```python
from build123d import *

# Parameters (mm, degrees)
F0_W     = 295.148
F0_H     = 402.59
F0_R     = 6.0071
F1_DEPTH = 2.54


with BuildPart() as f1:
    # F0 (on Front) → F1 (new body)
    with BuildSketch(Plane.XZ):
        with Locations((110.562274, -122.229906)):
            Rectangle(F0_W, F0_H)
        with Locations((-24.654626, -284.789906)):
            Circle(F0_R, mode=Mode.SUBTRACT)
        with BuildLine():
            Line((-30.661726, -258.754906), (4.898274, -258.754906))
            Line((4.898274, -258.754906), (4.898274, -310.824906))
            Line((4.898274, -310.824906), (-30.661726, -310.824906))
            Line((-30.661726, -310.824906), (-30.661726, -297.489906))
            Line((-30.661726, -297.489906), (-24.654626, -297.489906))
            ThreePointArc((-24.654626, -297.489906), (-11.954626, -284.789906), (-24.654626, -272.089906))
            Line((-24.654626, -272.089906), (-30.661726, -272.089906))
            Line((-30.661726, -272.089906), (-30.661726, -258.754906))
        make_face(mode=Mode.SUBTRACT)
        with Locations((-24.654626, -183.189906)):
            Circle(F0_R, mode=Mode.SUBTRACT)
        with BuildLine():
            Line((-30.661726, -157.154906), (4.898274, -157.154906))
            Line((4.898274, -157.154906), (4.898274, -209.224906))
            Line((4.898274, -209.224906), (-30.661726, -209.224906))
            Line((-30.661726, -209.224906), (-30.661726, -195.889906))
            Line((-30.661726, -195.889906), (-24.654626, -195.889906))
            ThreePointArc((-24.654626, -195.889906), (-11.954626, -183.189906), (-24.654626, -170.489906))
            Line((-24.654626, -170.489906), (-30.661726, -170.489906))
            Line((-30.661726, -170.489906), (-30.661726, -157.154906))
        make_face(mode=Mode.SUBTRACT)
        with BuildLine():
            Line((251.786274, -290.504906), (216.226274, -290.504906))
            Line((216.226274, -290.504906), (216.226274, -238.434906))
            Line((216.226274, -238.434906), (251.786274, -238.434906))
            Line((251.786274, -238.434906), (251.786274, -251.769906))
            Line((251.786274, -251.769906), (245.779174, -251.769906))
            ThreePointArc((245.779174, -251.769906), (233.079174, -264.469906), (245.779174, -277.169906))
            Line((245.779174, -277.169906), (251.786274, -277.169906))
            Line((251.786274, -277.169906), (251.786274, -290.504906))
        make_face(mode=Mode.SUBTRACT)
        with Locations((245.779174, -264.469906)):
            Circle(F0_R, mode=Mode.SUBTRACT)
        with BuildLine():
            Line((251.786274, -150.169906), (245.779174, -150.169906))
            ThreePointArc((245.779174, -150.169906), (233.079174, -162.869906), (245.779174, -175.569906))
            Line((245.779174, -175.569906), (251.786274, -175.569906))
            Line((251.786274, -175.569906), (251.786274, -188.904906))
            Line((251.786274, -188.904906), (216.226274, -188.904906))
            Line((216.226274, -188.904906), (216.226274, -136.834906))
            Line((216.226274, -136.834906), (251.786274, -136.834906))
            Line((251.786274, -136.834906), (251.786274, -150.169906))
        make_face(mode=Mode.SUBTRACT)
        with Locations((245.779174, -162.869906)):
            Circle(F0_R, mode=Mode.SUBTRACT)
        with Locations((-24.654626, -81.589906)):
            Circle(F0_R, mode=Mode.SUBTRACT)
        with BuildLine():
            Line((-30.661726, -55.554906), (4.898274, -55.554906))
            Line((4.898274, -55.554906), (4.898274, -107.624906))
            Line((4.898274, -107.624906), (-30.661726, -107.624906))
            Line((-30.661726, -107.624906), (-30.661726, -94.289906))
            Line((-30.661726, -94.289906), (-24.654626, -94.289906))
            ThreePointArc((-24.654626, -94.289906), (-11.954626, -81.589906), (-24.654626, -68.889906))
            Line((-24.654626, -68.889906), (-30.661726, -68.889906))
            Line((-30.661726, -68.889906), (-30.661726, -55.554906))
        make_face(mode=Mode.SUBTRACT)
        with Locations((-24.654626, 20.010094)):
            Circle(F0_R, mode=Mode.SUBTRACT)
        with BuildLine():
            Line((-30.661726, 32.710094), (-30.661726, 46.045094))
            Line((-30.661726, 46.045094), (4.898274, 46.045094))
            Line((4.898274, 46.045094), (4.898274, -6.024906))
            Line((4.898274, -6.024906), (-30.661726, -6.024906))
            Line((-30.661726, -6.024906), (-30.661726, 7.310094))
            Line((-30.661726, 7.310094), (-24.654626, 7.310094))
            ThreePointArc((-24.654626, 7.310094), (-11.954626, 20.010094), (-24.654626, 32.710094))
            Line((-24.654626, 32.710094), (-30.661726, 32.710094))
        make_face(mode=Mode.SUBTRACT)
        with BuildLine():
            Line((216.226274, -35.234906), (251.786274, -35.234906))
            Line((251.786274, -35.234906), (251.786274, -48.569906))
            Line((251.786274, -48.569906), (245.779174, -48.569906))
            ThreePointArc((245.779174, -48.569906), (233.079174, -61.269906), (245.779174, -73.969906))
            Line((245.779174, -73.969906), (251.786274, -73.969906))
            Line((251.786274, -73.969906), (251.786274, -87.304906))
            Line((251.786274, -87.304906), (216.226274, -87.304906))
            Line((216.226274, -87.304906), (216.226274, -35.234906))
        make_face(mode=Mode.SUBTRACT)
        with Locations((245.779174, -61.269906)):
            Circle(F0_R, mode=Mode.SUBTRACT)
        with BuildLine():
            Line((251.786274, 27.630094), (251.786274, 14.295094))
            Line((251.786274, 14.295094), (216.226274, 14.295094))
            Line((216.226274, 14.295094), (216.226274, 66.365094))
            Line((216.226274, 66.365094), (251.786274, 66.365094))
            Line((251.786274, 66.365094), (251.786274, 53.030094))
            Line((251.786274, 53.030094), (245.779174, 53.030094))
            ThreePointArc((245.779174, 53.030094), (233.079174, 40.330094), (245.779174, 27.630094))
            Line((245.779174, 27.630094), (251.786274, 27.630094))
        make_face(mode=Mode.SUBTRACT)
        with Locations((245.779174, 40.330094)):
            Circle(F0_R, mode=Mode.SUBTRACT)
    extrude(amount=F1_DEPTH)


solid = f1.part
```
Geometry check sheet. Reference: the model listing, model coordinates, mm. A direction names the side the tool comes from. Round coordinates to 2 decimals unless told otherwise and drop trailing zeros. Loops run counter-clockwise (first coordinate to the right, second up) from the corner with the lowest first, then second, coordinate; pieces in that order, holes last. Notation, with made-up numbers: M -32.75,-15.75 L 8.25,-15.75 A5 ccw 8.25,-11.75 Z; hole C 14.25,-4.5 d11. An arc over 180 degrees is marked long. Return JSON: item names as keys, results as strings. Group by question number.
(1) Section check A-A, the plane x = 227. Enter the section's corners in (y, z).
(2) Section check B-B, the plane y = -1.3. Give the number of separate pieces and of enclosed holes in the cut face, and give its area (3 significant figures).
(3) Set-up check for faces 1 (the face through (108, 0, -119)), 2 (the face through (233.082, -1.252, 40.609)): record each of +Z, -Z, +X, -X, +Y, -Y from which the full face is reachable in a straight line by a thin tool's end or side.
(4) Mould release check, pull along X, two halves, no side actions. Record for faces 3 (the face through (108, -2.54, -119)), 4 (the face through (-11.958, -1.252, -81.869)): pulls with the +X half, pulls with the -X half, needs draft (parallel to the pull), parting line crosses it, or undercut.
(5) Scan lines: line 1 along Z through (x, y) = (217, -2.1); line 2 along Z through (x, y) = (3.5, -1.8); line 3 along X through (y, z) = (-1.9, -265). Record each from-to range of solid material in increasing order. Write a range as [from, to].
Data:
{
 "1": {"outline": "M -2.54,-323.52 L 0,-323.52 L 0,-290.5 L -2.54,-290.5 Z; M -2.54,-238.43 L 0,-238.43 L 0,-188.9 L -2.54,-188.9 Z; M -2.54,-136.83 L 0,-136.83 L 0,-87.3 L -2.54,-87.3 Z; M -2.54,-35.23 L 0,-35.23 L 0,14.3 L -2.54,14.3 Z; M -2.54,66.37 L 0,66.37 L 0,79.07 L -2.54,79.07 Z"},
 "2": {"separate pieces": "1", "enclosed holes": "16", "area": "106,000 mm²"},
 "3": {"face 1": "+Z, -Z, +X, -X, +Y", "face 2": "+Y, -Y"},
 "4": {"face 3": "needs draft", "face 4": "undercut"},
 "5": {"line 1": "[-323.52, -290.5], [-238.43, -188.9], [-136.83, -87.3], [-35.23, 14.3], [66.37, 79.07]", "line 2": "[-323.52, -310.82], [-258.75, -209.22], [-157.15, -107.62], [-55.55, -6.02], [46.05, 79.07]", "line 3": "[-37.01, -30.66], [4.9, 216.23], [233.09, 239.8], [251.76, 258.14]"}
}
